Read the model definition and answer for the solid it produces. Units are mm, in the model's axes. Give positions to 0.01 mm unless a question says otherwise; leave off trailing zeros. Loops run counter-clockwise (first coordinate to the right, second up) from the corner with the lowest first, then second, coordinate; pieces in that order, holes last. Notation, with made-up numbers: (49.5, 5) - (53.5, 5) arc R24 ccw to (53.5, 39) - close; hole circle Ø1 at (-36, 79). An arc over 180 degrees is marked (long way). Use a Markdown table: item, result. Add a question column.
Item 1: A cutting plane is placed at C-C (z = -1.9). Determine the outline of the cut face in (x, y) (3 decimals), plus the area to 3 significant figures.
Item 2: A cutting plane is placed at B-B (z = -9.75). Determine the outline of the cut face in (x, y), plus the area to 3 significant figures.
Item 3: A cutting plane is placed at D-D (x = 0.1). Determine the outline of the cut face in (y, z) (3 decimals), plus the area to 3 significant figures.
Item 4: Consider probe 1 along Y at (x, z) = (0.2, -1.9) (3 decimals); probe 2 along Y at (x, z) = (0.2, -17.5); probe 3 along Z at (x, y) = (0.1, 8). Determine where each line is inside the solid, lowest interval first. Write a range as [from, to].
Item 5: A cutting plane is placed at A-A (y = -4). Determine the outline of the cut face in (x, z).
from build123d import *

# Parameters (mm, degrees)
SKETCH2_R           = 0.93
BOSS_EXTRUDE1_DEPTH = 0.3


with BuildPart() as part:
    # Sketch2 → Boss-Extrude1 (new body)
    with BuildSketch(Plane(origin=(0, 0, 0), x_dir=(0, 0, -1), z_dir=(1, 0, 0))):
        Polygon((0, 0), (0, -9.8), (24.8771, -9.8), (24.8771, 24.2), (4.2771, 24.2), (4.2771, 25.3), (0.6771, 25.3), (0.6771, 20.6), (21.2771, 20.6), (21.2771, -6.2), (3.6, -6.2), (3.6, 0), align=None)
        with Locations((1.9, -2.295)):
            Circle(SKETCH2_R, mode=Mode.SUBTRACT)
    extrude(amount=BOSS_EXTRUDE1_DEPTH)


solid = part.part
Geometry says:
| question | item | result |
|---|---|---|
| 1 | outline | (0, -9.8) - (0.3, -9.8) - (0.3, -3.225) - (0, -3.225) - close; (0, -1.365) - (0.3, -1.365) - (0.3, 0) - (0, 0) - close; (0, 20.6) - (0.3, 20.6) - (0.3, 25.3) - (0, 25.3) - close |
| 1 | area | 3.79 mm² |
| 2 | outline | (0, -9.8) - (0.3, -9.8) - (0.3, -6.2) - (0, -6.2) - close; (0, 20.6) - (0.3, 20.6) - (0.3, 24.2) - (0, 24.2) - close |
| 2 | area | 2.16 mm² |
| 3 | outline | (-9.8, -24.877) - (24.2, -24.877) - (24.2, -4.277) - (25.3, -4.277) - (25.3, -0.677) - (20.6, -0.677) - (20.6, -21.277) - (-6.2, -21.277) - (-6.2, -3.6) - (0, -3.6) - (0, 0) - (-9.8, 0) - close; hole circle Ø1.86 at (-2.295, -1.9) |
| 3 | area | 297 mm² |
| 4 | probe 1 | [-9.8, -3.225], [-1.365, 0], [20.6, 25.3] |
| 4 | probe 2 | [-9.8, -6.2], [20.6, 24.2] |
| 4 | probe 3 | [-24.88, -21.28] |
| 5 | outline | (0, -24.88) - (0.3, -24.88) - (0.3, -21.28) - (0, -21.28) - close; (0, -3.6) - (0.3, -3.6) - (0.3, 0) - (0, 0) - close |
